For this review, take the finished solid that the model builds, in its own axes (mm). Face numbers are marked on the shaded views. A direction names the side the tool comes from. Coordinates: 2 decimals unless noted, no trailing zeros. Write each loop counter-clockwise with the first axis right and the second up, starting at its lowest first coordinate (ties: lowest second). Pieces come first, ordered by that corner, then holes.
1) Mouldability with a two-part tool opening along Y and no side actions: class the marked faces 1, 2 and 3 as pulls with the +Y half, pulls with the -Y half, needs draft (parallel to the pull), parting line crosses it, or undercut.
2) We need section D-D on y = 4.75. Write out the cut boundary in (x, z).
3) Insertion check: P1, Ø2, axis at y = -4.5, z = 5, coming from the -X side; P2, Ø5, axis at y = -1.5, z = 4.5, coming from the -X side; P3, Ø3, axis at x = 6.5, y = -3.5, coming from the +Z side. Each pin has a flat end and moves straight along its axis. Give the tip position at first contact, or say it passes through.
4) For the marked faces 4 and 5, list the 3-axis set-ups (+Z, -Z, +X, -X, +Y, -Y) from which the entire face can be reached by the end or side of a thin tool; tool diameter is ignored.
5) To check wall thickness, follow line 1 along Y through (x, z) = (5.25, -3.5); line 2 along Z through (x, y) = (0, 0.75). State the ranges of each line that lie inside material, in increasing order.
6) We need section C-C on y = -2.25. Write out the cut boundary in (x, z).
from build123d import *


with BuildPart() as part:
    # Sketch2 → Revolve1 (revolve)
    with BuildSketch(Plane.XY):
        with BuildLine():
            Line((2.4967819, -5.588), (2.4967819, 5.588))
            Line((2.4967819, 5.588), (6.5024, 5.588))
            ThreePointArc((6.5024, 5.588), (8.001, 4.0894), (6.5024, 2.5908))
            Line((6.5024, 2.5908), (3.9751, 2.5908))
            Line((3.9751, 2.5908), (3.9751, -2.5908))
            Line((3.9751, -2.5908), (6.5024, -2.5908))
            ThreePointArc((6.5024, -2.5908), (8.001, -4.0894), (6.5024, -5.588))
            Line((6.5024, -5.588), (2.4967819, -5.588))
        make_face()
    revolve(axis=Axis((0, 0, 0), (0, 1, 0)))

    # Sketch3 → Cut-Revolve1 (revolve, cut)
    with BuildSketch(Plane.XY):
        Polygon((0, 5.588), (5.2197, 5.588), (2.5019, 2.286), (0, 2.286), align=None)
    revolve(axis=Axis((0, 2.286, 0), (0, 1, 0)), mode=Mode.SUBTRACT)


solid = part.part
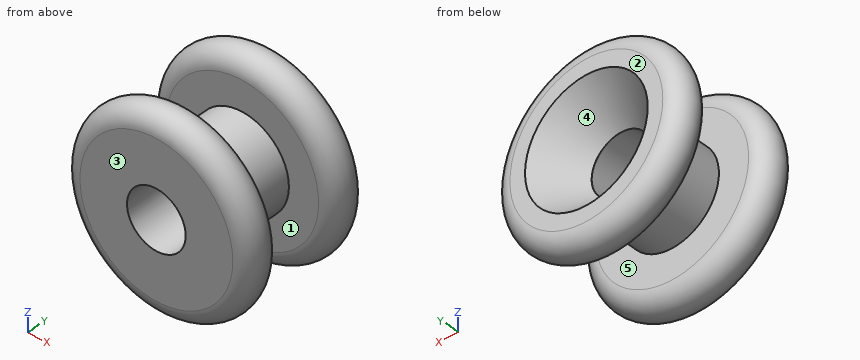
Result:
1. face 1: undercut
1. face 2: pulls with the +Y half
1. face 3: pulls with the -Y half
2. outline: circle Ø15.7 at (0, 0); hole circle Ø9.06 at (0, 0)
3. P1: stops at x = -6.9
3. P2: stops at x = -7.29
3. P3: stops at z = 6.19
4. face 4: +Y
4. face 5: none
5. line 1: y = -5.59 to -2.59, 2.59 to 5.59
5. line 2: z = -3.98 to -2.5, 2.5 to 3.98
6. outline: circle Ø7.95 at (0, 0); hole circle Ø4.99 at (0, 0)
